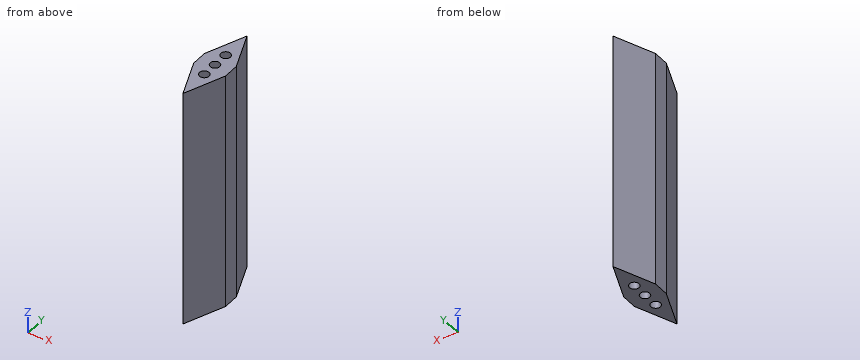
```python
from build123d import *

# Parameters (mm, degrees)
F0_W       = 20
F0_H       = 60
F1_DEPTH   = 150
F2_D       = 6
F2_DEPTH   = 150
F2_TIP     = 1.8025818571
F3_SIZE2   = 10
F3_SIZE    = 25
F3_2_SIZE2 = 9.99999
F3_2_SIZE  = 24.99999


# Not quite as in the source:
# - a fillet or chamfer is up to 0.001 mm smaller than in the source, because OpenCascade refuses the exact size


with BuildPart() as f1:
    # F0 (on Top) → F1 (new body)
    with BuildSketch(Plane.XY):
        Rectangle(F0_W, F0_H)
    extrude(amount=F1_DEPTH)

    # F2
    with Locations(Plane(origin=(0, 0, 0), x_dir=(1, 0, 0), z_dir=(0, 0, -1))):
        with Locations((0, -10), (0, 0), (0, 10)):
            Hole(F2_D / 2, depth=F2_DEPTH)
            with Locations((0, 0, -(F2_DEPTH + F2_TIP / 2))):  # 118° drill point
                Cone(0, F2_D / 2, F2_TIP, mode=Mode.SUBTRACT)

    # F3
    f3_edges = [f1.edges().sort_by_distance(p)[0] for p in [
        (-10, 30, 75),
        (-10, -30, 75),
    ]]
    f3_side = f1.faces().sort_by_distance((-10, 0, 75))[0]
    chamfer(f3_edges, length=F3_SIZE, length2=F3_SIZE2, reference=f3_side)

    # F3#2 (size 25 and 10 in the source; OpenCascade refuses exactly that, so slightly less here)
    f3_2_edges = [f1.edges().sort_by_distance(p)[0] for p in [
        (10, -30, 75),
        (10, 30, 75),
    ]]
    f3_2_side = f1.faces().sort_by_distance((10, 0, 75))[0]
    chamfer(f3_2_edges, length=F3_2_SIZE, length2=F3_2_SIZE2, reference=f3_2_side)


solid = f1.part
```
Geometry: final body of the model. Coordinates: model frame, mm. Round coordinates to 2 decimals unless told otherwise and drop trailing zeros. Write each loop counter-clockwise with the first axis right and the second up, starting at its lowest first coordinate (ties: lowest second). Pieces come first, ordered by that corner, then holes. Notation, with made-up numbers: M 73,7.25 L 98,7.25 A15 ccw 98,14.25 Z; hole C 66.25,-32.5 d7. An arc over 180 degrees is marked long. Answer in a Markdown table with one row per item. Add a question column.
(1) Cut plane C-C, the plane y = 0. Return the cut outline in (x, z), then the cut area to 3 significant figures.
(2) Cut plane A-A, the plane y = 10. Return the cut outline in (x, z), then the cut area to 3 significant figures.
(3) Contact query for flat-ended pins moving along their axis: pin 1 (6 mm diameter, centred on y = -18.5, z = 17.5, fed in from -X); pin 2 (2 mm diameter, centred on x = -7.5, z = 91.5, fed in from -Y); pin 3 (1.5 mm diameter, centred on x = 0, y = -2, fed in from -Z); pin 4 (3 mm diameter, centred on x = -2.5, z = 122, fed in from +Y). Output: stop coordinate, or through.
(4) Cut plane D-D, the plane y = 26.5. Return the cut outline in (x, z).
(5) Cut plane B-B, the plane z = 100.5. Give the number of separate pieces and of enclosed holes in the cut face, then the cut area to 3 significant figures.
(6) Ray query, L1, parallel to X at y = 10, z = 58.5; L2, parallel to X at y = -1, z = 39; L3, parallel to X at y = 15, z = 57.5. Return the intervals inside material, ascending.
Established:
| question | item | result |
|---|---|---|
| 1 | outline | M -10,0 L -3,0 L -3,150 L -10,150 Z; M 3,0 L 10,0 L 10,150 L 3,150 Z |
| 1 | area | 2,100 mm² |
| 2 | outline | M -8,0 L -3,0 L -3,150 L -8,150 Z; M 3,0 L 8,0 L 8,150 L 3,150 Z |
| 2 | area | 1,500 mm² |
| 3 | pin 1 | x = -5.8 |
| 3 | pin 2 | y = -13.75 |
| 3 | pin 3 | through |
| 3 | pin 4 | y = 27.5 |
| 4 | outline | M -1.4,0 L 1.4,0 L 1.4,150 L -1.4,150 Z |
| 5 | separate pieces | 1 |
| 5 | enclosed holes | 3 |
| 5 | area | 615 mm² |
| 6 | L1 | -8 to -3, 3 to 8 |
| 6 | L2 | -10 to -2.83, 2.83 to 10 |
| 6 | L3 | -6 to 6 |
